from build123d import *

# Parameters (mm, degrees)
BOSS_EXTRUDE1_DEPTH     = 2
SKETCH5_W               = 4
SKETCH5_H               = 2
CUT_EXTRUDE3_DEPTH      = 123
FILLET3_SIZE            = 4
FILLET3_SIZE_2          = 1.2
SKETCH6_W               = 5
SKETCH6_H               = 5
BOSS_EXTRUDE3_DEPTH     = 4
FILLET4_R               = 2.5
CUT_EXTRUDE7_DEPTH      = 23
CUT_EXTRUDE7_DEPTH_BACK = 10
SKETCH7_R               = 1.5
CUT_EXTRUDE8_DEPTH      = 103
CUT_EXTRUDE8_DEPTH_BACK = 10
SKETCH8_R               = 1.578894268
SKETCH11_W              = 5
SKETCH11_H              = 7.941397329
SKETCH11_W_2            = 5.025588604
SKETCH11_W_3            = 4.996681142
SKETCH11_W_4            = 5.000407309
CUT_EXTRUDE10_DEPTH     = 2
BOSS_EXTRUDE9_DEPTH     = 5
BOSS_EXTRUDE10_DEPTH    = 5


# Some blends are built 0.0001 mm under size
with BuildPart() as part:
    # Sketch1 → Boss-Extrude1 (new body)
    with BuildSketch(Plane(origin=(0, 0, 0), x_dir=(1, 0, 0), z_dir=(0, 1, 0))):
        with BuildLine():
            Line((-124.990139359, 1941.929047201), (-26.990139359, 1941.929047201))
            Line((-26.990139359, 1941.929047201), (-26.990139359, 1869.177480284))
            add(Edge.make_bspline(
                [(-26.990139359, 1869.177480284), (-26.971518988, 1862.10424426), (-30.008687271, 1852.889636427), (-37.937395583, 1843.840603399), (-46.643299948, 1837.427446423), (-55.223933615, 1835.160216105), (-61.011506847, 1835.177480284)],
                knots=[0, 0, 0, 0, 0.39690732, 0.518030206, 0.674278755, 1, 1, 1, 1], degree=3))
            Line((-61.011506847, 1835.177480284), (-91.011506847, 1835.177480284))
            add(Edge.make_bspline(
                [(-124.990139359, 1869.177480284), (-125.031653114, 1863.882416947), (-123.319081347, 1856.812557982), (-118.175654079, 1848.334494738), (-113.169582942, 1842.947577461), (-104.127691798, 1837.037384536), (-96.235416895, 1835.16563891), (-91.011506847, 1835.177480284)],
                knots=[0, 0, 0, 0, 0.297124953, 0.397302783, 0.556358073, 0.706503021, 1, 1, 1, 1], degree=3))
            Line((-124.990139359, 1869.177480284), (-124.990139359, 1941.929047201))
        make_face()
    extrude(amount=BOSS_EXTRUDE1_DEPTH)

    # Sketch5 → Cut-Extrude3 (cut)
    with BuildSketch(Plane(origin=(-26.990139359, 0, 0), x_dir=(0, 0, -1), z_dir=(1, 0, 0))):
        with Locations((1939.929047201, 1)):
            Rectangle(SKETCH5_W, SKETCH5_H)
    extrude(amount=-CUT_EXTRUDE3_DEPTH, mode=Mode.SUBTRACT)

    # Fillet3
    # an asymmetric fillet: 4, 1.2 mm, written as the material it takes off along each edge
    with BuildSketch(Plane(origin=(-16.990139359, 0, -1937.929047201), x_dir=(0, 0, 1), z_dir=(-1, 0, 0))) as fillet3_piece_1:
        with BuildLine():
            Bezier((FILLET3_SIZE, 0), (0, 0), (0, FILLET3_SIZE_2), weights=[1, 0.707106781, 1])
            Line((0, FILLET3_SIZE_2), (0, 0))
            Line((0, 0), (FILLET3_SIZE, 0))
        make_face()
    extrude(amount=118, mode=Mode.SUBTRACT)

    # Sketch6 → Boss-Extrude3 (add)
    with BuildSketch(Plane(origin=(0, 2, 0), x_dir=(1, 0, 0), z_dir=(0, 1, 0))):
        with Locations((-42.490139359, 1935.429047201)):
            Rectangle(SKETCH6_W, SKETCH6_H)
        with Locations((-109.490139359, 1935.429047201)):
            Rectangle(SKETCH6_W, SKETCH6_H)
    extrude(amount=BOSS_EXTRUDE3_DEPTH)

    # Fillet4
    fillet4_edges = [part.edges().sort_by_distance(p)[0] for p in [
        (-42.490139359, 6, -1932.929047201),
        (-42.490139359, 6, -1937.929047201),
        (-109.490139359, 6, -1932.929047201),
        (-109.490139359, 6, -1937.929047201),
    ]]
    fillet(fillet4_edges, radius=FILLET4_R - 0.0001)  # a hair under: the kernel refuses the full size

    # Sketch7 → Cut-Extrude7 (cut, two sides: drawn at the far end of the back side and taken through both)
    with BuildSketch(Plane.ZY.offset(111.990139359).offset(-CUT_EXTRUDE7_DEPTH_BACK)):
        with Locations(Location((-1935.429047201, 2.500019457, 0), (0, 0, 199.472008932))):
            Circle(SKETCH7_R)
    extrude(amount=CUT_EXTRUDE7_DEPTH + CUT_EXTRUDE7_DEPTH_BACK, mode=Mode.SUBTRACT)

    # Sketch8 → Cut-Extrude8 (cut, two sides: drawn at the far end of the back side and taken through both)
    with BuildSketch(Plane(origin=(-39.990139359, 0, 0), x_dir=(0, 0, -1), z_dir=(1, 0, 0)).offset(-CUT_EXTRUDE8_DEPTH_BACK)):
        with Locations(Location((1935.429047201, 2.421125189, 0), (0, 0, 195.469275058))):
            Circle(SKETCH8_R)
    extrude(amount=CUT_EXTRUDE8_DEPTH + CUT_EXTRUDE8_DEPTH_BACK, mode=Mode.SUBTRACT)

    # Sketch11 → Cut-Extrude10 (cut)
    with BuildSketch(Plane(origin=(0, 2, 0), x_dir=(1, 0, 0), z_dir=(0, 1, 0))):
        with Locations((-114.490139359, 1933.958348537)):
            Rectangle(SKETCH11_W, SKETCH11_H)
        with Locations((-104.477345057, 1933.958348537)):
            Rectangle(SKETCH11_W_2, SKETCH11_H)
        with Locations((-47.48847993, 1933.958348537)):
            Rectangle(SKETCH11_W_3, SKETCH11_H)
        with Locations((-37.489935704, 1933.958348537)):
            Rectangle(SKETCH11_W_4, SKETCH11_H)
    extrude(amount=-CUT_EXTRUDE10_DEPTH, mode=Mode.SUBTRACT)

    # Sketch12 → Boss-Extrude9 (add)
    with BuildSketch(Plane.ZY.offset(111.990139359)):
        with BuildLine():
            Line((-1924.299895593, 2), (-1934.170448036, 4.660075958))
            add(Edge.make_bspline(
                [(-1934.170448036, 4.660075958), (-1933.941696195, 4.343587233), (-1933.419980381, 3.982722954), (-1933.044506849, 2.985103355), (-1932.921466188, 2.346520539), (-1933.020256273, 1.890017898)],
                knots=[0, 0, 0, 0, 0.374528061, 0.57386245, 1, 1, 1, 1], degree=3))
            Line((-1933.020256273, 1.890017898), (-1924.299895593, 2))
        make_face()
    extrude(amount=-BOSS_EXTRUDE9_DEPTH)

    # Sketch13 → Boss-Extrude10 (add)
    with BuildSketch(Plane(origin=(-39.990139359, 0, 0), x_dir=(0, 0, -1), z_dir=(1, 0, 0))):
        Polygon((1933.084337522, 4.367373347), (1924.299895593, 2), (1933.057886548, 2), (1933.341968005, 3.330037979), (1934.06795395, 4.267766953), (1934.612443409, 4.7319029), align=None)
    extrude(amount=-BOSS_EXTRUDE10_DEPTH)


solid = part.part
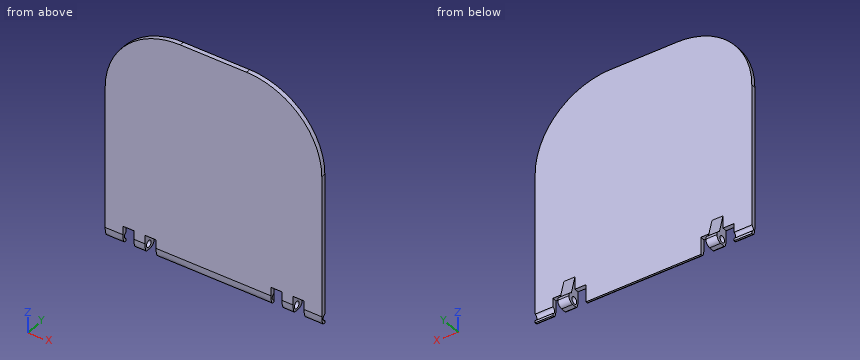
Check sheet for the modelled part. Datum: model origin and axes. Units: mm. Give positions to 0.01 mm unless a question says otherwise; leave off trailing zeros. Loops run counter-clockwise (first coordinate to the right, second up) from the corner with the lowest first, then second, coordinate; pieces in that order, holes last. Notation, with made-up numbers: M 4,-38 L 18,-38 A13 cw 18,-18 Z; hole C -26.75,-40 d11. An arc over 180 degrees is marked long. Use a Markdown table: item, result. Add a question column.
Q1. Sectioned sample at A-A, the plane z = -1905. Record the cut outline in (x, y), then the cut area to 3 significant figures.
Q2. Go/stop test with flat-tipped pins: pin 1 (2.5 mm diameter, centred on y = 2.5, z = -1935.43, fed in from -X); pin 2 (3 mm diameter, centred on y = 4.5, z = -1930, fed in from -X); pin 3 (1 mm diameter, centred on x = -105.5, y = 0.5, fed in from -Z). Record where each tip stops, or that it passes through.
Q3. Scan lines: line 1 along Y through (x, z) = (-69.5, -1910.5); line 2 along Z through (x, y) = (-109.5, 5.75); line 3 along X through (y, z) = (0.5, -1866). Record each from-to range of solid material in increasing order. Write a range as [from, to].
Verdict:
| question | item | result |
|---|---|---|
| 1 | outline | M -124.99,0 L -26.99,0 L -26.99,2 L -124.99,2 Z |
| 1 | area | 196 mm^2 |
| 2 | pin 1 | x = -101.96 |
| 2 | pin 2 | x = -111.99 |
| 2 | pin 3 | z = -1929.99 |
| 3 | line 1 | [0, 2] |
| 3 | line 2 | [-1936.52, -1934.34] |
| 3 | line 3 | [-124.86, -27.14] |
